Drawing for the job (mm, zero at the part's lowest x, y, z). A direction names the side the tool comes from. Round coordinates to 2 decimals unless told otherwise and drop trailing zeros. Loops run counter-clockwise (first coordinate to the right, second up) from the corner with the lowest first, then second, coordinate; pieces in that order, holes last. Notation, with made-up numbers: (6, 39) - (55, 39) arc R29 ccw to (55, 63) - close; hole circle Ø6 at (54.5, -18.5). An arc over 180 degrees is marked (long way). Put each result on its own line as item: value.
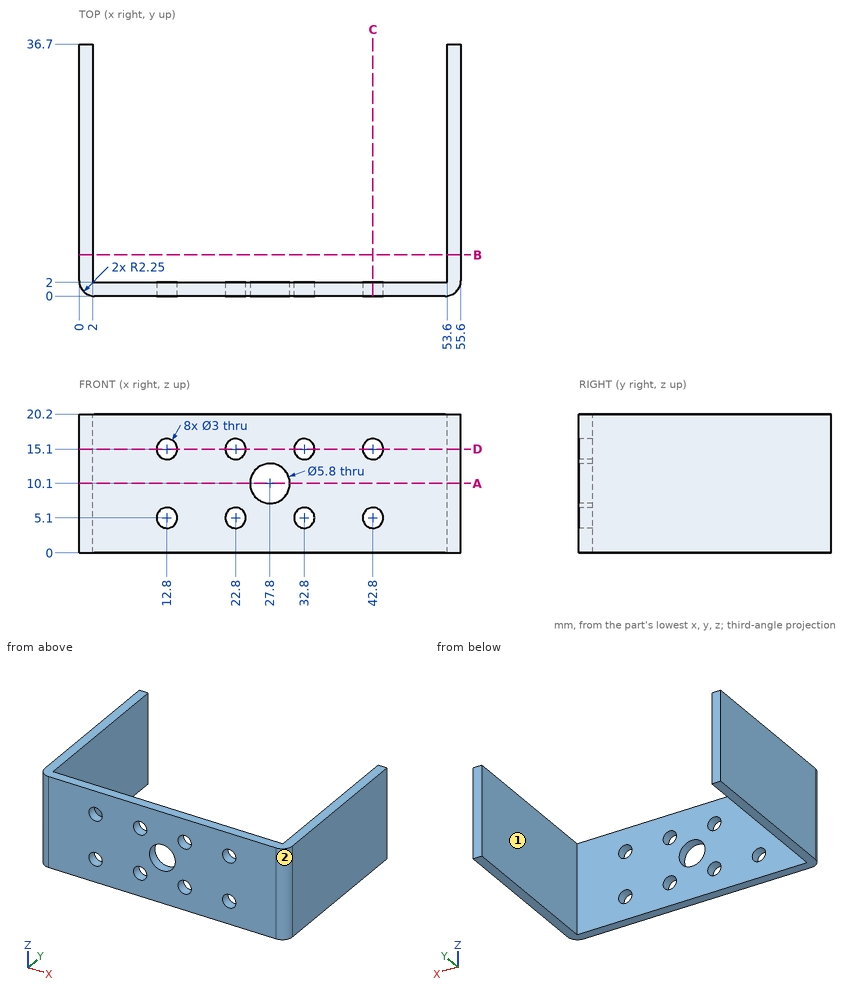
1. Band-saw the part on D-D (z = 15.1). List the corners of the cut face in (x, y).
A:
outline: (0, 2.25) arc R2.25 ccw to (2.25, 0) - (11.3, 0) - (11.3, 2) - (2, 2) - (2, 36.7) - (0, 36.7) - close; (14.3, 0) - (21.3, 0) - (21.3, 2) - (14.3, 2) - close; (24.3, 0) - (31.3, 0) - (31.3, 2) - (24.3, 2) - close; (34.3, 0) - (41.3, 0) - (41.3, 2) - (34.3, 2) - close; (44.3, 0) - (53.35, 0) arc R2.25 ccw to (55.6, 2.25) - (55.6, 36.7) - (53.6, 36.7) - (53.6, 2) - (44.3, 2) - close
2. Band-saw the part on C-C (x = 42.8). List the corners of the cut face in (y, z).
A:
outline: (0, 0) - (2, 0) - (2, 3.6) - (0, 3.6) - close; (0, 6.6) - (2, 6.6) - (2, 13.6) - (0, 13.6) - close; (0, 16.6) - (2, 16.6) - (2, 20.2) - (0, 20.2) - close
3. Band-saw the part on A-A (z = 10.1). List the corners of the cut face in (x, y).
A:
outline: (0, 2.25) arc R2.25 ccw to (2.25, 0) - (24.9, 0) - (24.9, 2) - (2, 2) - (2, 36.7) - (0, 36.7) - close; (30.7, 0) - (53.35, 0) arc R2.25 ccw to (55.6, 2.25) - (55.6, 36.7) - (53.6, 36.7) - (53.6, 2) - (30.7, 2) - close
4. Band-saw the part on B-B (y = 6). List the corners of the cut face in (x, z).
A:
outline: (0, 0) - (2, 0) - (2, 20.2) - (0, 20.2) - close; (53.6, 0) - (55.6, 0) - (55.6, 20.2) - (53.6, 20.2) - close
5. Tool access for the marked faces 1 and 2: list every direction of +Z, -Z, +X, -X, +Y, -Y with a clear straight run to the whole face (end or side of a thin tool).
A:
face 1: +Z, -Z, +Y
face 2: +Z, -Z, +X, -Y
6. Pin check, flat tips, straight feed: P1, Ø2.5, axis at x = 22.8, z = 15.1, coming from the -Y side; P2, Ø6, axis at x = 34.5, z = 14.5, coming from the +Y side. Stop position of each tip, or through.
A:
P1: passes through
P2: stops at y = 2
7. Probe line 1 along Z through (x, y) = (32.8, 0.65); line 2 along X through (y, z) = (4, 18.5); line 3 along Z through (x, y) = (22, 1). List the from-to ranges inside material, lowest first. Write a range as [from, to].
A:
line 1: z = [0, 3.6], [6.6, 13.6], [16.6, 20.2]
line 2: x = [0, 2], [53.6, 55.6]
line 3: z = [0, 3.83], [6.37, 13.83], [16.37, 20.2]
